Can you work these out from the model? Positions are in its coordinate system, mm. A direction names the side the tool comes from. Give positions to 0.01 mm unless a question says otherwise; leave off trailing zeros. Write each loop counter-clockwise with the first axis right and the second up, starting at its lowest first coordinate (ties: lowest second). Pieces come first, ordered by that corner, then holes. Notation, with made-up numbers: (61.5, -23) - (110.5, -23) arc R18 ccw to (110.5, 5) - close; hole circle Ø9 at (89, -26.5). An arc over 180 degrees is marked (long way). Return JSON: item names as keys, results as strings. Group by question number.
from build123d import *

# Parameters (mm, degrees)
F4_DEPTH = 122.3


with BuildPart() as f1:
    # F0 (on Front) → F1 (revolve)
    with BuildSketch(Plane.XZ):
        Polygon((-86.8375, 30), (-96.8375, 30), (-96.8375, 34), (-98.8375, 34), (-100.947656, 0), (-96.8375, 0), (-86.8375, 0), align=None)
    revolve(axis=Axis((0, 0, -4.859696), (0, 0, -1)))

    # F2 (on Front) + F3 (on Front) → F4 (cut)
    with BuildSketch(Plane.XZ):
        with BuildLine():
            Line((5, 34), (-5, 34))
            ThreePointArc((-5, 34), (0, 29), (5, 34))
        make_face()
    with BuildSketch(Plane.XZ):
        with BuildLine():
            Line((0, 0), (7.5, 0))
            ThreePointArc((7.5, 0), (0, 7.5), (-7.5, 0))
            Line((-7.5, 0), (0, 0))
        make_face()
    extrude(amount=F4_DEPTH, mode=Mode.SUBTRACT)


solid = f1.part
1) On a 3-axis mill with a long thin cutter (end or side, diameter ignored), from which of +Z, -Z, +X, -X, +Y, -Y can I reach the whole of each face in a straight line? I mean faces 1 (the face through (0, -94, 29)), 2 (the face through (0.16, -93.49, 7.5)), 3 (the face through (-40.07, -77.04, 15.21)). Say none if no direction works.
2) Imagine slicing it at A-A, the plane z = 20.5. Write out the boundary of the cut face in (x, y) (1 decimal), and give its area (3 significant figures).
3) We'd pull the mould along X, two halves only. Please class faces 4 (the face through (-58, 65, 30)), 5 (the face through (-44.4, 75.3, 0)), 6 (the face through (21.556, -97.074, 24.318)): pulls with the +X half, pulls with the -X half, needs draft (parallel to the pull), parting line crosses it, or undercut.
4) I need wall thicknesses on line 1 along X through (y, z) = (0, 33.1); line 2 along Y through (x, z) = (-57, 15.5); line 3 along X through (y, z) = (7, 32). Which ranges of each line are inside material? Lowest first, please.
5) Imagine slicing it at B-B, the plane z = 5. Write out the boundary of the cut face in (x, y) (1 decimal).
6) Will these pins go through, and if not, where does the flat tip stop? pin 1 Ø12 at (x, z) = (66, 29.5) entering from +Y; pin 2 Ø5 at (x, z) = (-70.5, 11) entering from +Y; pin 3 Ø6 at (y, z) = (14, 17.5) entering from +X.
Resolved:
{
 "1": {"face 1": "+Z, -Y", "face 2": "-Z, -Y", "face 3": "+Z, -Z"},
 "2": {"outline": "circle Ø199.4 at (0, 0); hole circle Ø173.7 at (0, 0)", "area": "7,520 mm^2"},
 "3": {"face 4": "undercut", "face 5": "needs draft", "face 6": "parting line crosses it"},
 "4": {"line 1": "-98.89 to -96.84, 96.84 to 98.89", "line 2": "-82.15 to -65.51, 65.51 to 82.15", "line 3": "-98.71 to -96.58, 96.58 to 98.71"},
 "5": {"outline": "(-5.6, -100.5) - (-5.6, -86.7) arc R86.8 cw (long way) to (5.6, -86.7) - (5.6, -100.5) arc R100.6 ccw (long way) to start"},
 "6": {"pin 1": "y = 78.92", "pin 2": "y = 73.69", "pin 3": "x = 99.3"}
}
